Design review of the part built by this model. Coordinates are the model's own, in mm. A direction names the side the tool comes from. Round coordinates to 2 decimals unless told otherwise and drop trailing zeros. Loops run counter-clockwise (first coordinate to the right, second up) from the corner with the lowest first, then second, coordinate; pieces in that order, holes last. Notation, with made-up numbers: M -12.5,42 L 13.5,42 A32 ccw 13.5,73 Z; hole C 23,-14 d11. An arc over 180 degrees is marked long. Use a Markdown table: item, result.
from build123d import *

# Parameters (mm, degrees)
SKETCH1_R                            = 40
BOSS_EXTRUDE1_DEPTH                  = 78
F_6_5_6_5_DIAMETER_HOLE1_D           = 6.5
MIRROR2_AT_THE_SECOND_PLANE_COPY_1_D = 6.5


with BuildPart() as part:
    # Sketch1 → Boss-Extrude1 (new body)
    with BuildSketch(Plane(origin=(0, 0, 0), x_dir=(1, 0, 0), z_dir=(0, 1, 0))):
        with BuildLine():
            Line((-74, 50), (-74, 35))
            Line((-74, 35), (-56, 35))
            Line((-56, 35), (-56, -30))
            Line((-56, -30), (-40, -30))
            ThreePointArc((-40, -30), (0, -50), (40, -30))
            Line((40, -30), (56, -30))
            Line((56, -30), (56, 35))
            Line((56, 35), (74, 35))
            Line((74, 35), (74, 50))
            Line((74, 50), (-74, 50))
        make_face()
        with Locations(Location((0, 0, 0), (0, 0, 270))):
            Circle(SKETCH1_R, mode=Mode.SUBTRACT)
    extrude(amount=BOSS_EXTRUDE1_DEPTH)

    # Ø6.5 (6.5) Diameter Hole1 (through all)
    with Locations(Plane(origin=(65, 69, -35), x_dir=(1, 0, 0), z_dir=(0, 0, 1))):
        with Locations((0, 0), (0, -9)):
            f_6_5_6_5_diameter_hole1 = Hole(F_6_5_6_5_DIAMETER_HOLE1_D / 2)

    # Mirror2: Ø6.5 (6.5) Diameter Hole1 across plane
    add(f_6_5_6_5_diameter_hole1.mirror(Plane.ZX.offset(39)), mode=Mode.SUBTRACT)

    # Mirror2 at the second plane: Ø6.5 (6.5) Diameter Hole1 across plane
    add(f_6_5_6_5_diameter_hole1.mirror(Plane(origin=(0, 0, 0), x_dir=(0, 0, 1), z_dir=(1, 0, 0))), mode=Mode.SUBTRACT)

    # Mirror2 at the second plane copy 1 (through all)
    with Locations(Plane(origin=(-65, 9, -35), x_dir=(-1, 0, 0), z_dir=(0, 0, 1))):
        with Locations((0, 0), (0, -9)):
            Hole(MIRROR2_AT_THE_SECOND_PLANE_COPY_1_D / 2)


solid = part.part
1. Machinability: for faces 5 (the face through (68.247, 8.857, -42.605)), 6 (the face through (-56, 38, -3)), 7 (the face through (65, 38, -35)), which of the approach directions +Z, -Z, +X, -X, +Y, -Y give a long, thin tool a straight path to every point of the face, cutting with its end or side? Answer none if there is none.
Check values:
| item | result |
|---|---|
| face 5 | +Z, -Z |
| face 6 | +Z, -X, +Y, -Y |
| face 7 | +Z, +X, +Y, -Y |
2. Insertion check: pin 1 (10.5 mm diameter, centred on x = -65, y = 69, fed in from -Z); pin 2 (5 mm diameter, centred on x = -50, y = 26.5, fed in from +Z); pin 3 (8 mm diameter, centred on x = 15.5, y = 31.5, fed in from +Z); pin 4 (1 mm diameter, centred on x = -27, y = 63.5, fed in from +Z). Each pin has a flat end and moves straight along its axis. Give the tip position at first contact, or say it passes through.
Check values:
| item | result |
|---|---|
| pin 1 | stops at z = -50 |
| pin 2 | stops at z = 30 |
| pin 3 | stops at z = 48.66 |
| pin 4 | stops at z = 42.4 |
3. Take a section at D-D on x = 65. Give the boundary of the cut face in (y, z), and give its area (3 significant figures).
Check values:
| item | result |
|---|---|
| outline | M 0,-50 L 5.75,-50 L 5.75,-35 L 0,-35 Z; M 12.25,-50 L 14.75,-50 L 14.75,-35 L 12.25,-35 Z; M 21.25,-50 L 56.75,-50 L 56.75,-35 L 21.25,-35 Z; M 63.25,-50 L 65.75,-50 L 65.75,-35 L 63.25,-35 Z; M 72.25,-50 L 78,-50 L 78,-35 L 72.25,-35 Z |
| area | 780 mm² |
4. Take a section at A-A on y = 60. Give the boundary of the cut face in (x, z).
Check values:
| item | result |
|---|---|
| outline | M -74,-50 L -68.25,-50 L -68.25,-35 L -74,-35 Z; M -61.75,-50 L 61.75,-50 L 61.75,-35 L 56,-35 L 56,30 L 40,30 A50 ccw -40,30 L -56,30 L -56,-35 L -61.75,-35 Z; M 68.25,-50 L 74,-50 L 74,-35 L 68.25,-35 Z; hole C 0,0 d80 |
5. Take a section at C-C on y = 49. Give the boundary of the cut face in (x, z).
Check values:
| item | result |
|---|---|
| outline | M -74,-50 L 74,-50 L 74,-35 L 56,-35 L 56,30 L 40,30 A50 ccw -40,30 L -56,30 L -56,-35 L -74,-35 Z; hole C 0,0 d80 |
6. Wall thickness on line 1 along Y through (x, z) = (65, -38); line 2 along Z through (x, y) = (61, 33); line 3 along Z through (x, y) = (-35, 54.5): over which ranges is each line inside the solid? List them lowest first. Write a range as from..to.
Check values:
| item | result |
|---|---|
| line 1 | y = 0..5.75, 12.25..14.75, 21.25..56.75, 63.25..65.75, 72.25..78 |
| line 2 | z = -50..-35 |
| line 3 | z = -50..-19.36, 19.36..35.71 |
7. The part is to be moulded in two halves that separate along X. For faces 1 (the face through (48, 38, 30)), 2 (the face through (-74, 38, -43)), 3 (the face through (-67.579, 67.022, -42.605)), 4 (the face through (74, 38, -42)), say which applies: pulls with the +X half, pulls with the -X half, needs draft (parallel to the pull), parting line crosses it, or undercut.
Check values:
| item | result |
|---|---|
| face 1 | needs draft |
| face 2 | pulls with the -X half |
| face 3 | undercut |
| face 4 | pulls with the +X half |
8. Take a section at B-B on x = 0. Give the boundary of the cut face in (y, z), and give its area (3 significant figures).
Check values:
| item | result |
|---|---|
| outline | M 0,-50 L 78,-50 L 78,-40 L 0,-40 Z; M 0,40 L 78,40 L 78,50 L 0,50 Z |
| area | 1,560 mm² |
